from build123d import *

# Parameters (mm, degrees)
SKETCH1_R           = 101.374642805
BOSS_EXTRUDE1_DEPTH = 6.35
CUT_EXTRUDE1_DEPTH  = 7.35


with BuildPart() as part:
    # Sketch1 → Boss-Extrude1 (new body)
    with BuildSketch(Plane(origin=(0, 0, 0), x_dir=(1, 0, 0), z_dir=(0, 1, 0))):
        Circle(SKETCH1_R)
    extrude(amount=BOSS_EXTRUDE1_DEPTH)

    # Sketch2 → Cut-Extrude1 (cut, through all)
    with BuildSketch(Plane(origin=(0, 6.35, 0), x_dir=(1, 0, 0), z_dir=(0, 1, 0))):
        with BuildLine():
            ThreePointArc((-101.374642805, 1.78e-07), (-101.174780653, -6.362543795), (-100.575982241, -12.7))
            Line((-100.575982241, -12.7), (-57.078868275, -12.7))
            Line((-57.078868275, -12.7), (-50.574642805, -12.7))
            Line((-50.574642805, -12.7), (-50.574642805, 12.7))
            Line((-50.574642805, 12.7), (-100.575982241, 12.7))
            ThreePointArc((-100.575982241, 12.7), (-101.174780642, 6.362543972), (-101.374642805, 1.78e-07))
        make_face()
        with BuildLine():
            ThreePointArc((2.49e-07, 101.374642805), (-6.36254376, 101.174780655), (-12.7, 100.575982241))
            Line((-12.7, 100.575982241), (-12.7, 57.078868275))
            Line((-12.7, 57.078868275), (-12.7, 50.574642805))
            Line((-12.7, 50.574642805), (12.7, 50.574642805))
            Line((12.7, 50.574642805), (12.7, 100.575982241))
            ThreePointArc((12.7, 100.575982241), (6.362544008, 101.17478064), (2.49e-07, 101.374642805))
        make_face()
        with BuildLine():
            Line((50.574642805, -12.7), (100.575982241, -12.7))
            ThreePointArc((100.575982241, -12.7), (101.174780648, -6.362543884), (101.374642805, 0))
            ThreePointArc((101.374642805, 0), (101.174780648, 6.362543884), (100.575982241, 12.7))
            Line((100.575982241, 12.7), (57.078868275, 12.7))
            Line((57.078868275, 12.7), (50.574642805, 12.7))
            Line((50.574642805, 12.7), (50.574642805, -12.7))
        make_face()
        with BuildLine():
            Line((12.7, -50.574642805), (-12.7, -50.574642805))
            Line((-12.7, -50.574642805), (-12.7, -100.575982241))
            ThreePointArc((-12.7, -100.575982241), (-6.362543952, -101.174780643), (-1.37e-07, -101.374642805))
            ThreePointArc((-1.37e-07, -101.374642805), (6.362543815, -101.174780652), (12.7, -100.575982241))
            Line((12.7, -100.575982241), (12.7, -57.078868275))
            Line((12.7, -57.078868275), (12.7, -50.574642805))
        make_face()
    extrude(amount=-CUT_EXTRUDE1_DEPTH, mode=Mode.SUBTRACT)


solid = part.part
Build history of the part. All positions in model axes, mm. A direction names the side the tool comes from. Coordinates: 2 decimals unless noted, no trailing zeros. Order: outer loops, then holes, each group sorted by start corner. A loop starts at its lowest first (then second) coordinate and runs counter-clockwise, first axis right, second up. Notation, with made-up numbers: (34.25, -36) - (38.25, -36) arc R15 ccw to (38.25, -23) - close; hole circle Ø5 at (-10, -9). An arc over 180 degrees is marked (long way). Write item = value, one per line. Start each with the question number.
1) Saw through at D-D on x = -8. Write the cut outline in (y, z).
2) Wall check: line 1 along X through (y, z) = (4.5, -4.5); line 2 along X through (y, z) = (5.5, -13); line 3 along X through (y, z) = (0.5, -69). Give the ranges that are in metal, low to high. Write a range as from..to.
3) Saw through at A-A on y = 3.25. Write the cut outline in (x, z), then the cut area to 3 significant figures.
4) Flat gauge pins, fed straight in: pin 1 Ø3 at (x, y) = (88, 4.5) entering from -Z; pin 2 Ø3 at (x, y) = (-28.5, 3) entering from +Z; pin 3 Ø3 at (y, z) = (2, 85) entering from +X. Where does each tip first touch, or does it go through?
5) 3-axis set-ups, long thin cutter, end or side, ignore diameter. For faces 1 (the face through (12.7, 3, -75)), 2 (the face through (76, 3, -12.7)), 3 (the face through (-12.7, 3, 75)): which of +Z, -Z, +X, -X, +Y, -Y reach the whole face in a straight line?
6) Saw through at B-B on z = 73.5. Write the cut outline in (x, y).
7) Saw through at C-C on x = 76. Write the cut outline in (y, z), then the cut area to 3 significant figures.
8) Two-plate mould, pull along X, no slides. Class faces 4 (the face through (-75, 3, -12.7)), 5 (the face through (50.575, 3, 0)), 6 (the face through (-12.7, 3, -76)): pulls with the +X half, pulls with the -X half, needs draft (parallel to the pull), parting line crosses it, or undercut.
From the geometry:
q1.outline = (0, -50.57) - (6.35, -50.57) - (6.35, 50.57) - (0, 50.57) - close
q2.line_1 = -50.57..50.57
q2.line_2 = -100.54..100.54
q2.line_3 = -74.27..-12.7, 12.7..74.27
q3.outline = (-100.58, -12.7) arc R101.37 ccw to (-12.7, -100.58) - (-12.7, -50.57) - (12.7, -50.57) - (12.7, -100.58) arc R101.37 ccw to (100.58, -12.7) - (50.57, -12.7) - (50.57, 12.7) - (100.58, 12.7) arc R101.37 ccw to (12.7, 100.58) - (12.7, 50.57) - (-12.7, 50.57) - (-12.7, 100.58) arc R101.37 ccw to (-100.58, 12.7) - (-50.57, 12.7) - (-50.57, -12.7) - close
q3.area = 27,200 mm^2
q4.pin_1 = -52.86
q4.pin_2 = 97.71
q4.pin_3 = 57.49
q5.face_1 = -Z, +Y, -Y
q5.face_2 = +X, +Y, -Y
q5.face_3 = +Z, +Y, -Y
q6.outline = (-69.82, 0) - (-12.7, 0) - (-12.7, 6.35) - (-69.82, 6.35) - close; (12.7, 0) - (69.82, 0) - (69.82, 6.35) - (12.7, 6.35) - close
q7.outline = (0, -67.09) - (6.35, -67.09) - (6.35, -12.7) - (0, -12.7) - close; (0, 12.7) - (6.35, 12.7) - (6.35, 67.09) - (0, 67.09) - close
q7.area = 691 mm^2
q8.face_4 = needs draft
q8.face_5 = pulls with the +X half
q8.face_6 = undercut
